Source: CAD feature listing. Evaluate the final solid. Frame: model axes, mm. A direction names the side the tool comes from. Coordinates: 2 decimals unless noted, no trailing zeros. Loops run counter-clockwise (first coordinate to the right, second up) from the corner with the lowest first, then second, coordinate; pieces in that order, holes last.
Item 1: Pull-direction query (X, two-part tool) for faces 3 (the cylindrical face through (11.62, 29.05, 1.75)), 4 (the cylindrical face through (0, 0.6, 1.7)), 5 (the flat face through (0, 38, 0)); classes: +X half, -X half, draft (parallel to the pull), parting line (faces both ways), or undercut.
Item 2: Section query A-A, the plane z = 0.7. Return the cut outline in (x, y).
Item 3: Section query C-C, the plane x = 12.5. Return the cut outline in (y, z).
Item 4: Pin query (flat end, axial travel): pin 1 Ø1 at (y, z) = (16.5, 2) entering from +X; pin 2 Ø1.7 at (x, y) = (0, 33.5) entering from +Z; pin 3 Ø1.5 at (x, z) = (-3, 1.5) entering from -Y. Return the tip coordinate at first contact, or that it passes through.
Item 5: Section query B-B, the plane y = 26. Return the cut outline in (x, z), then the cut area to 3 significant figures.
Item 6: Reachability of faces 1 (the cylindrical face through (-2.81, 39.21, 1.75)), 2 (the flat face through (-25, 47, 2)) from +Z, -Z, +X, -X, +Y, -Y: full face, straight path, thin tool, end or side. Return the list, or none.
Item 7: Line query: probe 1 along X at (y, z) = (21, 1.55); probe 2 along X at (y, z) = (67, 2.95); probe 3 along Z at (x, y) = (-14, 61). Output: solid intervals per line, ascending.
Item 8: Section query D-D, the plane y = 34. Return the cut outline in (x, z), then the cut area to 3 significant figures.
```python
from build123d import *

# Parameters (mm, degrees)
EXTRUDE_1_DEPTH     = 2
EXTRUDE_2_DEPTH     = 1.5
OTHER_START         = 1.5
OTHER_1_DEPTH       = 0.5
CUT_EXTRUDE_1_DEPTH = 10


# Read off the part's stored shape, not the designer's step: Полость1
with BuildPart() as part:
    # Эскиз1 → Бобышка-Вытянуть1 (new body)
    with BuildSketch(Plane.XY):
        with BuildLine():
            Line((-2.248831138, 1.132455321), (-19.497662275, 9.818536847))
            ThreePointArc((-19.497662275, 9.818536847), (-23.514006776, 13.504841411), (-25, 18.75))
            Line((-25, 18.75), (-25, 75))
            Line((-25, 75), (25, 75))
            Line((25, 75), (25, 18.75))
            ThreePointArc((25, 18.75), (23.514006776, 13.504841411), (19.497662275, 9.818536847))
            Line((19.497662275, 9.818536847), (2.248831138, 1.132455321))
            ThreePointArc((2.248831138, 1.132455321), (0, 0.598186897), (-2.248831138, 1.132455321))
        make_face()
    extrude(amount=EXTRUDE_1_DEPTH)

    # Эскиз2 → Бобышка-Вытянуть2 (add)
    with BuildSketch(Plane.XY.offset(2)):
        with BuildLine():
            Line((25, 75), (-25, 75))
            Line((-25, 75), (-25, 18.75))
            ThreePointArc((-25, 18.75), (-23.514006776, 13.504841411), (-19.497662275, 9.818536847))
            Line((-19.497662275, 9.818536847), (-2.248831138, 1.132455321))
            ThreePointArc((-2.248831138, 1.132455321), (0, 0.598186897), (2.248831138, 1.132455321))
            Line((2.248831138, 1.132455321), (19.497662275, 9.818536847))
            ThreePointArc((19.497662275, 9.818536847), (23.514006776, 13.504841411), (25, 18.75))
            Line((25, 18.75), (25, 75))
        make_face()
        with BuildLine():
            Line((23, 73), (-23, 73))
            Line((-23, 73), (-23, 18.75))
            ThreePointArc((-23, 18.75), (-21.81120542, 14.553873129), (-18.59812982, 11.604829477))
            Line((-18.59812982, 11.604829477), (-1.349298683, 2.918747951))
            ThreePointArc((-1.349298683, 2.918747951), (0, 2.598186897), (1.349298683, 2.918747951))
            Line((1.349298683, 2.918747951), (18.59812982, 11.604829477))
            ThreePointArc((18.59812982, 11.604829477), (21.81120542, 14.553873129), (23, 18.75))
            Line((23, 18.75), (23, 73))
        make_face(mode=Mode.SUBTRACT)
    extrude(amount=EXTRUDE_2_DEPTH)

    # Полость1 outline → Полость1 (cut)
    with BuildSketch(Plane.XY.offset(OTHER_START)):
        with BuildLine():
            ThreePointArc((5.872817683, 36.335212556), (10.497140141, 33.683878279), (5.659180925, 31.446003782))
            ThreePointArc((5.659180925, 31.446003782), (2.557547726, 38.996194393), (1.5, 47.089840022))
            Line((1.5, 47.089840022), (2.25, 61.864840022))
            ThreePointArc((2.25, 61.864840022), (1.66872912, 65.046820537), (0, 67.817780472))
            ThreePointArc((0, 67.817780472), (-1.66872912, 65.046820537), (-2.25, 61.864840022))
            Line((-2.25, 61.864840022), (-1.5, 47.089840022))
            ThreePointArc((-1.5, 47.089840022), (-2.557547726, 38.996194393), (-5.659180925, 31.446003782))
            ThreePointArc((-5.659180925, 31.446003782), (-10.49714014, 33.683878279), (-5.872817683, 36.335212556))
            Line((-5.872817683, 36.335212556), (-6.73484174, 48.66273089))
            ThreePointArc((-6.73484174, 48.66273089), (-10.164455559, 58.47909234), (-18, 65.314840022))
            Line((-18, 65.314840022), (-18, 20.314840022))
            Line((-18, 20.314840022), (-8.27498074, 20.314840022))
            ThreePointArc((-8.27498074, 20.314840022), (-6.018005307, 14.531627185), (-1.78373039, 9.991758821))
            ThreePointArc((-1.78373039, 9.991758821), (-0.762703724, 9.010745514), (0, 7.817780472))
            ThreePointArc((0, 7.817780472), (0.762703724, 9.010745514), (1.78373039, 9.991758821))
            ThreePointArc((1.78373039, 9.991758821), (6.018005307, 14.531627185), (8.27498074, 20.314840022))
            Line((8.27498074, 20.314840022), (18, 20.314840022))
            Line((18, 20.314840022), (18, 65.314840022))
            ThreePointArc((18, 65.314840022), (10.164455559, 58.47909234), (6.73484174, 48.66273089))
            Line((6.73484174, 48.66273089), (5.872817683, 36.335212556))
        make_face()
        with BuildLine():
            ThreePointArc((-1.5, 13.673911644), (-3.833724688, 16.727440499), (-5.212446581, 20.314840022))
            Line((-5.212446581, 20.314840022), (-1.5, 20.314840022))
            Line((-1.5, 20.314840022), (-1.5, 13.673911644))
        make_face(mode=Mode.SUBTRACT)
        with BuildLine():
            ThreePointArc((-7.92032189, 27.82958067), (-8.391822285, 25.594060154), (-8.55, 23.314840022))
            Line((-8.55, 23.314840022), (-15, 23.314840022))
            Line((-15, 23.314840022), (-15, 32.314840022))
            Line((-15, 32.314840022), (-13.309475019, 32.314840022))
            ThreePointArc((-13.309475019, 32.314840022), (-11.338226185, 29.203113691), (-7.92032189, 27.82958067))
        make_face(mode=Mode.SUBTRACT)
        with BuildLine():
            ThreePointArc((-4.896666667, 27.463714033), (-2.35750881, 26.043942439), (-1.35, 23.314840022))
            Line((-1.35, 23.314840022), (-5.55, 23.314840022))
            ThreePointArc((-5.55, 23.314840022), (-5.385666463, 25.414840022), (-4.896666667, 27.463714033))
        make_face(mode=Mode.SUBTRACT)
        with BuildLine():
            Line((1.5, 13.673911644), (1.5, 20.314840022))
            Line((1.5, 20.314840022), (5.212446581, 20.314840022))
            ThreePointArc((5.212446581, 20.314840022), (3.833724688, 16.727440499), (1.5, 13.673911644))
        make_face(mode=Mode.SUBTRACT)
        with BuildLine():
            ThreePointArc((1.35, 23.314840022), (2.35750881, 26.043942439), (4.896666667, 27.463714033))
            ThreePointArc((4.896666667, 27.463714033), (5.385666463, 25.414840022), (5.55, 23.314840022))
            Line((5.55, 23.314840022), (1.35, 23.314840022))
        make_face(mode=Mode.SUBTRACT)
        with BuildLine():
            ThreePointArc((0, 38.259555712), (1.403302974, 34.104361284), (3.327405339, 30.163202817))
            ThreePointArc((3.327405339, 30.163202817), (1.502516133, 29.26949151), (0, 27.901505478))
            ThreePointArc((0, 27.901505478), (-1.502516133, 29.26949151), (-3.327405339, 30.163202817))
            ThreePointArc((-3.327405339, 30.163202817), (-1.403302974, 34.104361284), (0, 38.259555712))
        make_face(mode=Mode.SUBTRACT)
        with BuildLine():
            ThreePointArc((8.55, 23.314840022), (8.391822285, 25.594060154), (7.92032189, 27.82958067))
            ThreePointArc((7.92032189, 27.82958067), (11.338226185, 29.203113691), (13.309475019, 32.314840022))
            Line((13.309475019, 32.314840022), (15, 32.314840022))
            Line((15, 32.314840022), (15, 23.314840022))
            Line((15, 23.314840022), (8.55, 23.314840022))
        make_face(mode=Mode.SUBTRACT)
        with BuildLine():
            ThreePointArc((-9.108112452, 39.595322211), (-11.782030233, 38.017722019), (-13.309475019, 35.314840022))
            Line((-13.309475019, 35.314840022), (-15, 35.314840022))
            Line((-15, 35.314840022), (-15, 59.587599146))
            ThreePointArc((-15, 59.587599146), (-11.277427711, 54.369586152), (-9.706680997, 48.155251207))
            Line((-9.706680997, 48.155251207), (-9.108112452, 39.595322211))
        make_face(mode=Mode.SUBTRACT)
        with BuildLine():
            ThreePointArc((9.706680998, 48.155251207), (11.277427711, 54.369586152), (15, 59.587599146))
            Line((15, 59.587599146), (15, 35.314840022))
            Line((15, 35.314840022), (13.309475019, 35.314840022))
            ThreePointArc((13.309475019, 35.314840022), (11.782030233, 38.017722019), (9.108112452, 39.595322211))
            Line((9.108112452, 39.595322211), (9.706680998, 48.155251207))
        make_face(mode=Mode.SUBTRACT)
    extrude(amount=OTHER_1_DEPTH, mode=Mode.SUBTRACT)

    # Эскиз3 → Вырез-Вытянуть1 (cut)
    with BuildSketch(Plane.XY.offset(1.5)):
        with BuildLine():
            Line((-18.3, 65.79134502), (-18.3, 20.014840022))
            Line((-18.3, 20.014840022), (-8.522704696, 20.014840022))
            ThreePointArc((-8.522704696, 20.014840022), (-6.205709985, 14.267416366), (-1.962700971, 9.75097776))
            ThreePointArc((-1.962700971, 9.75097776), (-0.776140503, 8.53640523), (0, 7.026200576))
            ThreePointArc((0, 7.026200576), (0.776140503, 8.53640523), (1.962700971, 9.75097776))
            ThreePointArc((1.962700971, 9.75097776), (6.205709985, 14.267416366), (8.522704696, 20.014840022))
            Line((8.522704696, 20.014840022), (18.3, 20.014840022))
            Line((18.3, 20.014840022), (18.3, 65.79134502))
            ThreePointArc((18.3, 65.79134502), (10.051283209, 58.844723617), (6.435652247, 48.684797911))
            Line((6.435652247, 48.684797911), (5.524546517, 35.655378948))
            ThreePointArc((5.524546517, 35.655378948), (10.188878559, 34.059650346), (5.889417806, 31.647808643))
            ThreePointArc((5.889417806, 31.647808643), (2.840648904, 39.098998924), (1.800000924, 47.0822489))
            Line((1.800000924, 47.0822489), (2.549996836, 61.857168373))
            ThreePointArc((2.549996836, 61.857168373), (1.8904299, 65.304748617), (0, 68.262300456))
            ThreePointArc((0, 68.262300456), (-1.8904299, 65.304748617), (-2.549996836, 61.857168373))
            Line((-2.549996836, 61.857168373), (-1.800000923, 47.0822489))
            ThreePointArc((-1.800000923, 47.0822489), (-2.840648904, 39.098998924), (-5.889417806, 31.647808643))
            ThreePointArc((-5.889417806, 31.647808643), (-10.188878559, 34.059650346), (-5.524546517, 35.655378948))
            Line((-5.524546517, 35.655378948), (-6.435652247, 48.684797911))
            ThreePointArc((-6.435652247, 48.684797911), (-10.051283209, 58.844723617), (-18.3, 65.79134502))
        make_face()
        with BuildLine():
            Line((-14.7, 58.862618748), (-14.7, 35.614840022))
            Line((-14.7, 35.614840022), (-13.537383539, 35.614840022))
            ThreePointArc((-13.537383539, 35.614840022), (-12.000472829, 38.223438928), (-9.424123799, 39.813818902))
            Line((-9.424123799, 39.813818902), (-10.006037257, 48.13556906))
            ThreePointArc((-10.006037257, 48.13556906), (-11.401876329, 53.915296555), (-14.7, 58.862618748))
        make_face(mode=Mode.SUBTRACT)
        with BuildLine():
            Line((10.006037257, 48.13556906), (9.424123799, 39.813818902))
            ThreePointArc((9.424123799, 39.813818902), (12.000472829, 38.223438928), (13.537383539, 35.614840022))
            Line((13.537383539, 35.614840022), (14.7, 35.614840022))
            Line((14.7, 35.614840022), (14.7, 58.862618748))
            ThreePointArc((14.7, 58.862618748), (11.401876329, 53.915296555), (10.006037257, 48.13556906))
        make_face(mode=Mode.SUBTRACT)
        with BuildLine():
            Line((8.847321215, 23.614840022), (14.7, 23.614840022))
            Line((14.7, 23.614840022), (14.7, 32.014840022))
            Line((14.7, 32.014840022), (13.537383539, 32.014840022))
            ThreePointArc((13.537383539, 32.014840022), (11.579925154, 29.014401424), (8.303170174, 27.566246767))
            ThreePointArc((8.303170174, 27.566246767), (8.692930904, 25.606749909), (8.847321215, 23.614840022))
        make_face(mode=Mode.SUBTRACT)
        with BuildLine():
            Line((-5.246590469, 23.614840022), (-1.661555581, 23.614840022))
            ThreePointArc((-1.661555581, 23.614840022), (-2.599333734, 25.86504954), (-4.69, 27.118837919))
            ThreePointArc((-4.69, 27.118837919), (-5.086558291, 25.385624396), (-5.246590469, 23.614840022))
        make_face(mode=Mode.SUBTRACT)
        with BuildLine():
            Line((1.661555581, 23.614840022), (5.246590469, 23.614840022))
            ThreePointArc((5.246590469, 23.614840022), (5.086558291, 25.385624396), (4.69, 27.118837919))
            ThreePointArc((4.69, 27.118837919), (2.599333734, 25.86504954), (1.661555581, 23.614840022))
        make_face(mode=Mode.SUBTRACT)
        with BuildLine():
            Line((-1.8, 20.014840022), (-4.830845042, 20.014840022))
            ThreePointArc((-4.830845042, 20.014840022), (-3.657955571, 17.030306032), (-1.8, 14.416666052))
            Line((-1.8, 14.416666052), (-1.8, 20.014840022))
        make_face(mode=Mode.SUBTRACT)
        with BuildLine():
            Line((4.830845043, 20.014840022), (1.8, 20.014840022))
            Line((1.8, 20.014840022), (1.8, 14.416666052))
            ThreePointArc((1.8, 14.416666052), (3.657955571, 17.030306032), (4.830845043, 20.014840022))
        make_face(mode=Mode.SUBTRACT)
        with BuildLine():
            Line((-13.537383539, 32.014840022), (-14.7, 32.014840022))
            Line((-14.7, 32.014840022), (-14.7, 23.614840022))
            Line((-14.7, 23.614840022), (-8.847321215, 23.614840022))
            ThreePointArc((-8.847321215, 23.614840022), (-8.692930904, 25.606749909), (-8.303170174, 27.566246767))
            ThreePointArc((-8.303170174, 27.566246767), (-11.579925154, 29.014401424), (-13.537383539, 32.014840022))
        make_face(mode=Mode.SUBTRACT)
        with BuildLine():
            ThreePointArc((2.89047704, 30.327467035), (1.328934128, 29.514243453), (0, 28.359391538))
            ThreePointArc((0, 28.359391538), (-1.328934128, 29.514243453), (-2.89047704, 30.327467035))
            ThreePointArc((-2.89047704, 30.327467035), (-1.260735073, 33.666741166), (0, 37.162074866))
            ThreePointArc((0, 37.162074866), (1.260735073, 33.666741166), (2.89047704, 30.327467035))
        make_face(mode=Mode.SUBTRACT)
    extrude(amount=CUT_EXTRUDE_1_DEPTH, mode=Mode.SUBTRACT)


solid = part.part
```
Verdict:
1. face 3: undercut
1. face 4: parting line
1. face 5: draft
2. outline: (-25, 18.75) arc R10 ccw to (-19.5, 9.82) - (-2.25, 1.13) arc R5 ccw to (2.25, 1.13) - (19.5, 9.82) arc R10 ccw to (25, 18.75) - (25, 75) - (-25, 75) - close
3. outline: (6.29, 0) - (75, 0) - (75, 3.5) - (73, 3.5) - (73, 2) - (61.76, 2) - (61.76, 1.5) - (56.01, 1.5) - (56.01, 2) - (37.65, 2) - (37.65, 1.5) - (29.98, 1.5) - (29.98, 2) - (23.61, 2) - (23.61, 1.5) - (20.01, 1.5) - (20.01, 2) - (8.53, 2) - (8.53, 3.5) - (6.29, 3.5) - close
4. pin 1: stops at x = 24.85
4. pin 2: stops at z = 2
4. pin 3: stops at y = 1.13
5. outline: (-25, 0) - (25, 0) - (25, 3.5) - (23, 3.5) - (23, 2) - (18.3, 2) - (18.3, 1.5) - (14.7, 1.5) - (14.7, 2) - (8.63, 2) - (8.63, 1.5) - (4.97, 1.5) - (4.97, 2) - (2.72, 2) - (2.72, 1.5) - (-2.72, 1.5) - (-2.72, 2) - (-4.97, 2) - (-4.97, 1.5) - (-8.63, 1.5) - (-8.63, 2) - (-14.7, 2) - (-14.7, 1.5) - (-18.3, 1.5) - (-18.3, 2) - (-23, 2) - (-23, 3.5) - (-25, 3.5) - close
5. area: 96.0 mm2
6. face 1: +Z
6. face 2: +Z, -Z, -X, +Y, -Y
7. probe 1: x = -25 to -18.3, 18.3 to 25
7. probe 2: x = -25 to -23, 23 to 25
7. probe 3: z = 0 to 1.5
8. outline: (-25, 0) - (25, 0) - (25, 3.5) - (23, 3.5) - (23, 2) - (18.3, 2) - (18.3, 1.5) - (10.19, 1.5) - (10.19, 2) - (4.68, 2) - (4.68, 1.5) - (1.12, 1.5) - (1.12, 2) - (-1.12, 2) - (-1.12, 1.5) - (-4.68, 1.5) - (-4.68, 2) - (-10.19, 2) - (-10.19, 1.5) - (-18.3, 1.5) - (-18.3, 2) - (-23, 2) - (-23, 3.5) - (-25, 3.5) - close
8. area: 94.3 mm2
